Could you check a few things on this model? Use its own coordinates, in mm. Face numbers are marked on the shaded views. A direction names the side the tool comes from. Coordinates: 2 decimals unless noted, no trailing zeros. Write each loop counter-clockwise with the first axis right and the second up, starting at its lowest first coordinate (ties: lowest second). Pieces come first, ordered by that corner, then holes. Notation, with made-up numbers: M -8,86 L 35,86 A23 ccw 35,116 Z; hole C 63,-21 d2. An arc over 180 degrees is marked long. Answer as CSV lines item,"result". Start each with the question number.
Item 1: Suppose I cut it at D-D, the plane z = 68.5. Write out the boundary of the cut face in (x, y), and give its area (3 significant figures).
Item 2: If I drill on line 1 along Y through (x, z) = (0, 1.1); line 2 along Z through (x, y) = (3.5, 7); line 3 along X through (y, z) = (3, 0.6), over which ranges is the centre line in solid material (lowest first)? Write a range as [from, to].
Item 3: Suppose I cut it at A-A, the plane y = 3. Write out the boundary of the cut face in (x, z).
Item 4: On a 3-axis mill with a long thin cutter (end or side, diameter ignored), from which of +Z, -Z, +X, -X, +Y, -Y can I reach the whole of each face in a straight line? I mean the marked faces 1, 2 and 3. Say none if no direction works.
Item 5: Suppose I cut it at B-B, the plane x = 0. Write out the boundary of the cut face in (y, z), and give its area (3 significant figures).
Item 6: I'm going to push flat-ended pins straight in: P1, Ø4, axis at x = 6, z = 45, coming from the +Y side; P2, Ø3, axis at x = -0.5, z = 56.5, coming from the -Y side; P3, Ø8, axis at y = 4.5, z = 48.5, coming from the +X side; P4, Ø3, axis at x = 6, z = 54, coming from the -Y side. Where does each tip first touch, or does it pass through?
Item 7: Suppose I cut it at C-C, the plane x = 4. Write out the boundary of the cut face in (y, z).
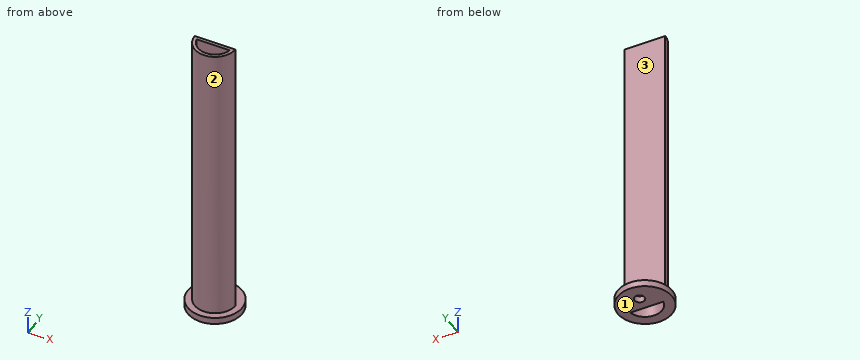
```python
from build123d import *

# Parameters (mm, degrees)
F1_DEPTH = 87
F0_R     = 8
F2_DEPTH = 2
F3_R     = 1.5
F4_DEPTH = 25


with BuildPart() as f1:
    # F0 (on Top) → F1 (new body)
    with BuildSketch(Plane.XY):
        with BuildLine():
            Line((6, 0), (-6, 0))
            ThreePointArc((-6, 0), (0, -6), (6, 0))
        make_face()
        with BuildLine():
            ThreePointArc((4.898979, -1), (0, -5), (-4.898979, -1))
            Line((-4.898979, -1), (4.898979, -1))
        make_face(mode=Mode.SUBTRACT)
    extrude(amount=F1_DEPTH)

    # F0 (on Top) → F2 (join)
    with BuildSketch(Plane.XY):
        Circle(F0_R)
        with BuildLine():
            ThreePointArc((6, 0), (0, -6), (-6, 0))
            Line((-6, 0), (6, 0))
        make_face(mode=Mode.SUBTRACT)
    extrude(amount=F2_DEPTH)

    # F3 (on face) → F4 (cut)
    with BuildSketch(Plane(origin=(0, 0, 0), x_dir=(1, 0, 0), z_dir=(0, 0, -1))):
        with Locations((0, -3)):
            Circle(F3_R)
    extrude(amount=-F4_DEPTH, mode=Mode.SUBTRACT)


solid = f1.part
```
Ans:
1,outline,"M -6,0 A6 ccw 6,0 Z; hole M -4.9,-1 A5 ccw 4.9,-1 Z"
1,area,"27.2 mm^2"
2,line 1,"y = [-8, -5], [-1, 1.5], [4.5, 8]"
2,line 2,"z = [0, 2]"
2,line 3,"x = [-7.42, -1.5], [1.5, 7.42]"
3,outline,"M -7.42,0 L -1.5,0 L -1.5,2 L -7.42,2 Z; M 1.5,0 L 7.42,0 L 7.42,2 L 1.5,2 Z"
4,face 1,"-Z, +X, -X, +Y, -Y"
4,face 2,"+Z, -Y"
4,face 3,"+Z, +X, -X, +Y"
5,outline,"M -8,0 L -5,0 L -5,87 L -6,87 L -6,2 L -8,2 Z; M -1,0 L 1.5,0 L 1.5,2 L 0,2 L 0,87 L -1,87 Z; M 4.5,0 L 8,0 L 8,2 L 4.5,2 Z"
5,area,"188 mm^2"
6,P1,"stops at y = 0"
6,P2,"stops at y = -6"
6,P3,"passes through"
6,P4,"stops at y = -3.97"
7,outline,"M -6.93,0 L -3,0 L -3,87 L -4.47,87 L -4.47,2 L -6.93,2 Z; M -1,0 L 6.93,0 L 6.93,2 L 0,2 L 0,87 L -1,87 Z"
